Part print with two shaded views. Sizes in mm from the minimum x, y, z corner. Coordinates: 2 decimals unless noted, no trailing zeros. Loops run counter-clockwise (first coordinate to the right, second up) from the corner with the lowest first, then second, coordinate; pieces in that order, holes last. Notation, with made-up numbers: (40, -15) -> (64, -15) arc R20 ccw to (64, 6) -> close; hole circle Ø7 at (-20.5, 64). An arc over 180 degrees is marked (long way). Return JSON: item names as keys, results as strings. Group by question number.
(1) Saw through at C-C on z = 2.05. Write the cut outline in (x, y) (3 decimals), then the cut area to 3 significant figures.
(2) Saw through at B-B on x = 173.99. Write the cut outline in (y, z) (3 decimals).
(3) Saw through at A-A on y = 62.01. Write the cut outline in (x, z) (3 decimals), then the cut area to 4 significant figures.
(4) Saw through at D-D on x = 41. Write the cut outline in (y, z), then the cut area to 3 significant figures.
(5) Probe L1, parallel to Y at x = 173.99, z = 1.75 (3 decimals); L2, parallel to Y at x = 15, z = 2.05; L3, parallel to X at y = 152.5, z = 2. List the from-to ranges inside material, lowest first.
(6) Flat gauge pins, fed straight in: pin 1 Ø9 at (x, y) = (173.99, 19.005) entering from -Z; pin 2 Ø1.5 at (x, z) = (11, 1.5) entering from +Y; pin 3 Ø0.9 at (y, z) = (194.5, 1.5) entering from +X; pin 4 Ø0.9 at (x, z) = (224, 1) entering from +Y (3 decimals). Where does each tip first touch, or does it go through?
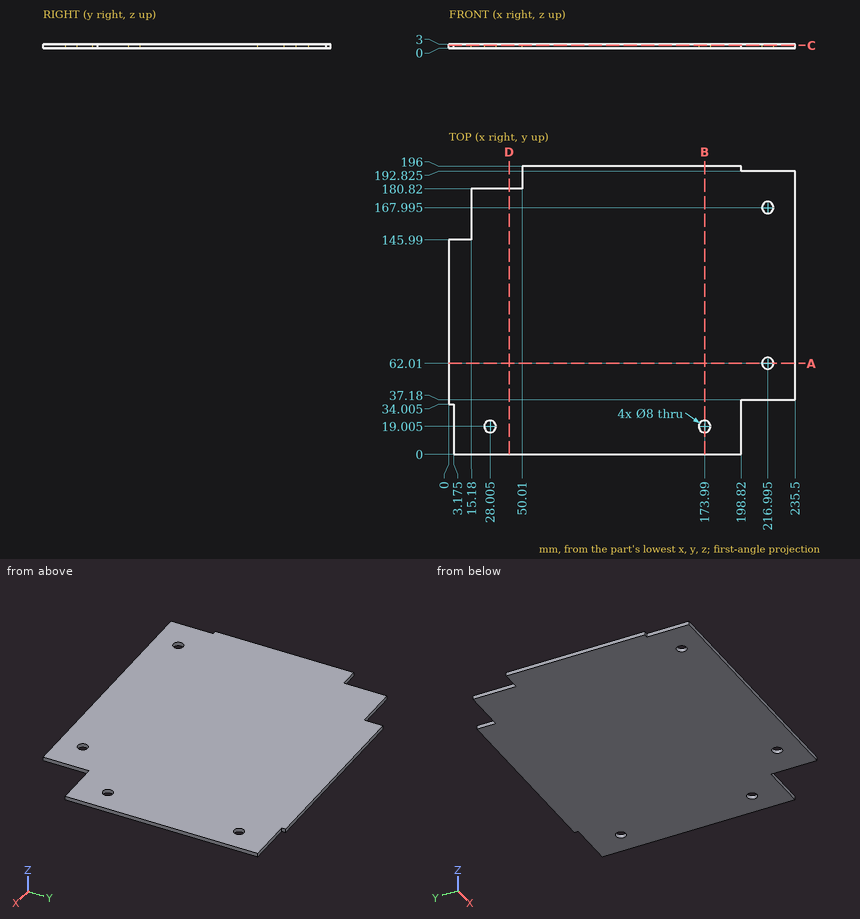
Geometry results:
{
 "1": {"outline": "(0, 34.005) -> (3.175, 34.005) -> (3.175, 0) -> (198.82, 0) -> (198.82, 37.18) -> (235.5, 37.18) -> (235.5, 192.825) -> (198.82, 192.825) -> (198.82, 196) -> (50.01, 196) -> (50.01, 180.82) -> (15.18, 180.82) -> (15.18, 145.99) -> (0, 145.99) -> close; hole circle Ø8 at (28.005, 19.005); hole circle Ø8 at (173.99, 19.005); hole circle Ø8 at (216.995, 62.01); hole circle Ø8 at (216.995, 167.995)", "area": "43,100 mm²"},
 "2": {"outline": "(0, 0) -> (15.005, 0) -> (15.005, 3) -> (0, 3) -> close; (23.005, 0) -> (196, 0) -> (196, 3) -> (23.005, 3) -> close"},
 "3": {"outline": "(0, 0) -> (212.995, 0) -> (212.995, 3) -> (0, 3) -> close; (220.995, 0) -> (235.5, 0) -> (235.5, 3) -> (220.995, 3) -> close", "area": "682.5 mm²"},
 "4": {"outline": "(0, 0) -> (180.82, 0) -> (180.82, 3) -> (0, 3) -> close", "area": "542 mm²"},
 "5": {"L1": "0 to 15.005, 23.005 to 196", "L2": "0 to 145.99", "L3": "15.18 to 235.5"},
 "6": {"pin 1": "z = 0", "pin 2": "y = 145.99", "pin 3": "x = 198.82", "pin 4": "y = 192.825"}
}
